Read the model definition and answer for the solid it produces. Units are mm, in the model's axes. Coordinates: 2 decimals unless noted, no trailing zeros. Loops run counter-clockwise (first coordinate to the right, second up) from the corner with the lowest first, then second, coordinate; pieces in that order, holes last.
Q1. Flat-ended cylindrical pins translate along their axes: P1, Ø4, axis at x = -25.84, z = -43.8, coming from the -Y side; P2, Ø1.5, axis at x = -49, y = 2, coming from the -Z side. Find the tip coordinate at first contact, or state that the pin passes through.
Q2. The mould has two halves that part along Z. Classify faces 1 (the face through (-60, 1, 1)), 2 (the face through (-20.253, 1.521, 13.579)), 3 (the face through (15, 1, 55.25)): pulls with the +Z half, pulls with the -Z half, needs draft (parallel to the pull), parting line crosses it, or undercut.
Q3. Section C-C (y = 2.3) is taken. Count the separate pieces of the cut face and the enclosed holes in it, then the cut area to 3 significant figures.
Q4. Straight lines are drawn through the part: line 1 (Z direction, x = 36.5, y = 0.85); line 2 (X direction, y = 1.65, z = -49.5); line 3 (X direction, y = 1.7, z = 17.5). For each, find the intervals that lie inside material, in ascending order.
Q5. Section A-A (x = -36.52) is taken. Give the vertices of the cut face in (y, z).
Q6. Section B-B (x = 26.5) is taken. Give the vertices of the cut face in (y, z).
Autodesk Inventor part; units mm, degrees
ref_plane "YZ Plane" through (0, 0, 0) normal (1, 0, 0) x (0, 1, 0)
ref_plane "XZ Plane" through (0, 0, 0) normal (0, 1, 0) x (-1, 0, 0)
ref_plane "XY Plane" through (0, 0, 0) normal (0, 0, 1) x (1, 0, 0)
sketch "Эскиз1" plane through (0, 0, 0) normal (0, 1, 0) x (-1, 0, 0)
  line L0 (-60, 55.25) -> (60, 55.25)
  line L1 (60, 55.25) -> (60, -55.25)
  line L2 (60, -55.25) -> (-60, -55.25)
  line L3 (-60, -55.25) -> (-60, 55.25)
  line L4 (60, -55.25) -> (-60, 55.25) construction
  point P0 (0, 0)
  point P1 (0, 0)
  dimension "d0" = 120
  dimension "d1" = 110.5
extrude "Выдавливание1" add sketch "Эскиз1" along normal blind 3
sketch "Эскиз2" plane through (0, 3, 0) normal (0, 1, 0) x (1, 0, 0)
  line L0 (-60, 55.25) -> (60, 55.25)
  line L1 (-60, 55.25) -> (-32, 55.25)
  line L2 (-32, 55.25) -> (-32, 47.25)
  line L3 (-32, 47.25) -> (-60, 47.25)
  line L4 (-60, 47.25) -> (-60, 55.25)
  line L5 (-60, -55.25) -> (-60, 55.25)
  line L6 (-60, -55.25) -> (-32, -55.25)
  line L7 (-32, -55.25) -> (-32, -47.25)
  line L8 (-32, -47.25) -> (-60, -47.25)
  line L9 (-60, -47.25) -> (-60, -55.25)
  point P0 (-60, -47.25)
  dimension "d12" = 28
  dimension "d13" = 8
  dimension "d14" = 28
  dimension "d15" = 8
extrude "Выдавливание2" cut sketch "Эскиз2" against normal blind 10
fillet "Сопряжение2" radius 2 8 edges at (-60, 1.5, 47.25) (-32, 1.5, 47.25) (-32, 1.5, 55.25) (-60, 1.5, -47.25) (-32, 1.5, -47.25) (-32, 1.5, -55.25) (60, 1.5, -55.25) (60, 1.5, 55.25)
sketch "Эскиз3" plane through (0, 3, 0) normal (0, 1, 0) x (1, 0, 0)
  circle A0 centre (-21.5, -13.0622) radius 1.35
  circle A1 centre (-21.5, 35.9378) radius 1.35
  circle A2 centre (36.5, 35.9378) radius 1.35
  circle A3 centre (36.5, -13.0622) radius 1.35
  line L0 (36.5, 25.9378) -> (-21.5, 25.9378) construction
  line L1 (-21.5, 25.9378) -> (-21.5, -23.0622) construction
  line L2 (-21.5, -23.0622) -> (36.5, -23.0622) construction
  line L3 (36.5, -23.0622) -> (36.5, 25.9378) construction
  circle A4 centre (36.5, -23.0622) radius 1.35
  circle A5 centre (36.5, 25.9378) radius 1.35
  circle A6 centre (-21.5, 25.9378) radius 1.35
  circle A7 centre (-21.5, -23.0622) radius 1.35
  line L4 (26.5, 35.9378) -> (-31.5, 35.9378) construction
  line L5 (-31.5, 35.9378) -> (-31.5, -13.0622) construction
  line L6 (-31.5, -13.0622) -> (26.5, -13.0622) construction
  line L7 (26.5, -13.0622) -> (26.5, 35.9378) construction
  circle A8 centre (-31.5, 35.9378) radius 1.35
  circle A9 centre (-31.5, -13.0622) radius 1.35
  circle A10 centre (26.5, -13.0622) radius 1.35
  circle A11 centre (26.5, 35.9378) radius 1.35
  line L8 (26.5, -23.0622) -> (-31.5, -23.0622) construction
  line L9 (-31.5, -23.0622) -> (-31.5, 25.9378) construction
  line L10 (-31.5, 25.9378) -> (26.5, 25.9378)
  line L11 (26.5, 25.9378) -> (26.5, -23.0622) construction
  circle A12 centre (26.5, 25.9378) radius 1.35
  circle A13 centre (26.5, -23.0622) radius 1.35
  circle A14 centre (-31.5, 25.9378) radius 1.35
  circle A15 centre (-31.5, -23.0622) radius 1.35
  point P0 (0, 0)
  dimension "d17" = 58
  dimension "d18" = 49
  dimension "d19" = 10
  dimension "d20" = 58
  dimension "d21" = 49
  dimension "d22" = 10
  dimension "d23" = 2.7
  dimension "d24" = 2.7
  dimension "d25" = 2.7
  dimension "d27" = 58
  dimension "d28" = 49
  dimension "d29" = 2.7
  dimension "d30" = 2.7
  dimension "d31" = 2.7
  dimension "d32" = 2.7
extrude "Выдавливание3" cut sketch "Эскиз3" against normal blind 10
sketch "Эскиз4" plane through (0, 3, 0) normal (0, 1, 0) x (1, 0, 0)
  circle A0 centre (-30.17, -18.3745) radius 1.5875
  circle A1 centre (-36.52, 29.8855) radius 1.5875
  circle A2 centre (46.03, 29.8855) radius 1.5875
  circle A3 centre (44.76, -18.3745) radius 1.5875
  point P0 (0, 0)
extrude "Выдавливание4" cut sketch "Эскиз4" against normal blind 10
sketch "Эскиз5" plane through (0, 3, 0) normal (0, 1, 0) x (1, 0, 0)
  point P0 (0, 0)
sketch "Эскиз6" plane through (0, 3, 0) normal (0, 1, 0) x (1, 0, 0)
  circle A0 centre (-25.8393, -31.2041) radius 1.45
  line L0 (-25.8393, -31.2041) -> (2.1607, -31.2041) construction
  line L1 (30.1607, -31.2041) -> (30.1607, 43.7959) construction
  line L2 (30.1607, 43.7959) -> (2.1607, 43.7959) construction
  line L3 (-25.8393, 43.7959) -> (-25.8393, -31.2041) construction
  circle A1 centre (30.1607, -31.2041) radius 1.45
  circle A2 centre (2.1607, -31.2041) radius 1.45
  circle A3 centre (30.1607, 6.2959) radius 1.45
  circle A4 centre (30.1607, 43.7959) radius 1.45
  circle A5 centre (-25.8393, 43.7959) radius 1.45
  circle A6 centre (2.1607, 43.7959) radius 1.45
  circle A7 centre (-25.8393, 6.2959) radius 1.45
  circle A8 centre (2.1607, 6.2959) radius 1.45
  line L4 (2.1607, 43.7959) -> (-25.8393, 43.7959) construction
  line L5 (2.1607, -31.2041) -> (30.1607, -31.2041) construction
  circle A9 centre (16.1607, -31.2041) radius 1.45
  circle A10 centre (-11.8393, -31.2041) radius 1.45
  circle A11 centre (-11.8393, 43.7959) radius 1.45
  circle A12 centre (16.1607, 43.7959) radius 1.45
  line L6 (2.1607, 43.7959) -> (2.1607, 6.2959) construction
  line L7 (2.1607, 6.2959) -> (2.1607, -31.2041) construction
  circle A13 centre (2.1607, -12.4541) radius 1.45
  circle A14 centre (2.1607, 25.0459) radius 1.45
  point P0 (0, 0)
  dimension "d37" = 2.9
  dimension "d38" = 56
  dimension "d39" = 75
  dimension "d40" = 2.9
  dimension "d41" = 2.9
extrude "Выдавливание5" cut sketch "Эскиз6" against normal blind 10
properties part number "фанера"
Numbers:
1. P1: stops at y = 0
1. P2: stops at z = -47.25
2. face 1: needs draft
2. face 2: undercut
2. face 3: pulls with the +Z half
3. separate pieces: 1
3. enclosed holes: 35
3. area: 12,600 mm2
4. line 1: z = -55.25 to -37.29, -34.59 to -27.29, -24.59 to 11.71, 14.41 to 21.71, 24.41 to 55.25
4. line 2: x = -32 to 60
4. line 3: x = -60 to -31.49, -28.85 to 43.44, 46.08 to 60
5. outline: (0, -47.25) - (3, -47.25) - (3, -31.47) - (0, -31.47) - close; (0, -28.3) - (3, -28.3) - (3, 47.25) - (0, 47.25) - close
6. outline: (0, -55.25) - (3, -55.25) - (3, -37.29) - (0, -37.29) - close; (0, -34.59) - (3, -34.59) - (3, -27.29) - (0, -27.29) - close; (0, -24.59) - (3, -24.59) - (3, 11.71) - (0, 11.71) - close; (0, 14.41) - (3, 14.41) - (3, 21.71) - (0, 21.71) - close; (0, 24.41) - (3, 24.41) - (3, 55.25) - (0, 55.25) - close
